CAD build for the part. Positions are in the model's coordinates, mm. Face numbers are marked on the shaded views. A direction names the side the tool comes from. Round coordinates to 2 decimals unless told otherwise and drop trailing zeros. Write each loop counter-clockwise with the first axis right and the second up, starting at its lowest first coordinate (ties: lowest second). Pieces come first, ordered by that corner, then holes. Notation, with made-up numbers: (51.5, 66) - (66.5, 66) arc R29 cw to (66.5, 90) - close; hole circle Ø8 at (13, 1). An arc over 180 degrees is marked (long way). Answer in a Markdown table with one row per item.
```python
from build123d import *

# Parameters (mm, degrees)
SKETCH1_W           = 20
SKETCH1_H           = 27
SKETCH1_R           = 2.5
BOSS_EXTRUDE1_DEPTH = 3
SKETCH2_W           = 3
SKETCH2_H           = 27
BOSS_EXTRUDE2_DEPTH = 15
SKETCH3_R           = 4
CUT_EXTRUDE1_DEPTH  = 15
CHAMFER1_SIZE       = 2


with BuildPart() as part:
    # Sketch1 → Boss-Extrude1 (new body)
    with BuildSketch(Plane(origin=(0, 0, 0), x_dir=(0, 0, -1), z_dir=(1, 0, 0))):
        with Locations((10, 13.5)):
            Rectangle(SKETCH1_W, SKETCH1_H)
        with Locations((10, 7)):
            Circle(SKETCH1_R, mode=Mode.SUBTRACT)
        with Locations((10, 20)):
            Circle(SKETCH1_R, mode=Mode.SUBTRACT)
    extrude(amount=BOSS_EXTRUDE1_DEPTH)

    # Sketch2 → Boss-Extrude2 (add)
    with BuildSketch(Plane(origin=(3, 0, 0), x_dir=(0, 0, -1), z_dir=(1, 0, 0))):
        with Locations((18.5, 13.5)):
            Rectangle(SKETCH2_W, SKETCH2_H)
    extrude(amount=BOSS_EXTRUDE2_DEPTH)

    # Sketch3 → Cut-Extrude1 (cut)
    with BuildSketch(Plane(origin=(0, 0, -20), x_dir=(-1, 0, 0), z_dir=(0, 0, -1))):
        with Locations((-10.5, 19.75)):
            Circle(SKETCH3_R)
        with Locations((-10.5, 7.25)):
            Circle(SKETCH3_R)
    extrude(amount=-CUT_EXTRUDE1_DEPTH, mode=Mode.SUBTRACT)

    # Chamfer1
    chamfer1_edges = [part.edges().sort_by_distance(p)[0] for p in [
        (18, 27, -18.5),
        (18, 0, -18.5),
    ]]
    chamfer(chamfer1_edges, length=CHAMFER1_SIZE)


solid = part.part
```
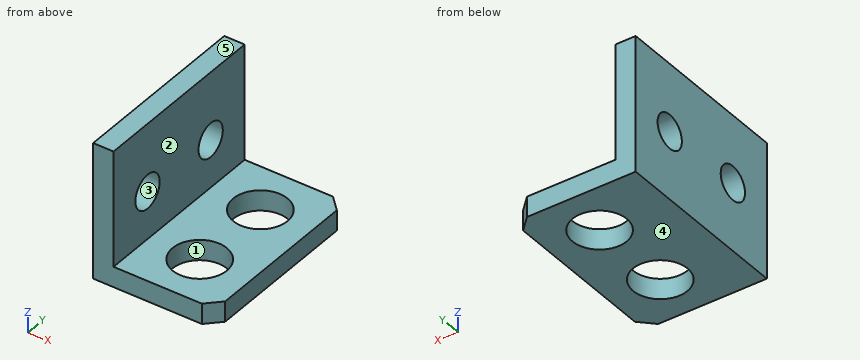
Q1. Saw through at C-C on z = -18.5. List the corners of the cut face in (x, y).
Computed:
| item | result |
|---|---|
| outline | (0, 0) - (16, 0) - (18, 2) - (18, 25) - (16, 27) - (0, 27) - close; hole circle Ø8 at (10.5, 7.25); hole circle Ø8 at (10.5, 19.75) |
Q2. Drill centre lines: line 1 (Y direction, x = 0.6, z = -10); line 2 (Y direction, x = 10.5, z = -18.15); line 3 (X direction, y = 21.25, z = -15). Where is each one in solid material? Low to high.
Computed:
| item | result |
|---|---|
| line 1 | y = 0 to 4.5, 9.5 to 17.5, 22.5 to 27 |
| line 2 | y = 0 to 3.25, 11.25 to 15.75, 23.75 to 27 |
| line 3 | x = 0 to 3 |
Q3. Saw through at B-B on x = 1.5. List the corners of the cut face in (y, z).
Computed:
| item | result |
|---|---|
| outline | (0, -20) - (27, -20) - (27, 0) - (0, 0) - close; hole circle Ø5 at (7, -10); hole circle Ø5 at (20, -10) |
Q4. 3-axis set-ups, long thin cutter, end or side, ignore diameter. For the marked faces 1 and 2: which of +Z, -Z, +X, -X, +Y, -Y reach the whole face in a straight line?
Computed:
| item | result |
|---|---|
| face 1 | +Z, -Z |
| face 2 | +Z, +X, +Y, -Y |
Q5. Flat gauge pins, fed straight in: pin 1 (8.5 mm diameter, centred on y = 17.5, z = -8, fed in from +X); pin 2 (5 mm diameter, centred on x = 15.5, y = 4.5, fed in from +Z). Where does each tip first touch, or does it go through?
Computed:
| item | result |
|---|---|
| pin 1 | stops at x = 3 |
| pin 2 | stops at z = -17 |
Q6. Saw through at D-D on x = 10.5. List the corners of the cut face in (y, z), then the cut area to 3 significant figures.
Computed:
| item | result |
|---|---|
| outline | (0, -20) - (3.25, -20) - (3.25, -17) - (0, -17) - close; (11.25, -20) - (15.75, -20) - (15.75, -17) - (11.25, -17) - close; (23.75, -20) - (27, -20) - (27, -17) - (23.75, -17) - close |
| area | 33.0 mm2 |
Q7. Pull direction Z, two halves, no side cores. Call the marked faces 3, 4 and 5: released by +Z, released by -Z, zero draft, split by the parting line, or undercut.
Computed:
| item | result |
|---|---|
| face 3 | undercut |
| face 4 | released by -Z |
| face 5 | released by +Z |
Q8. Saw through at A-A on z = -12. List the corners of the cut face in (x, y).
Computed:
| item | result |
|---|---|
| outline | (0, 0) - (3, 0) - (3, 5.5) - (0, 5.5) - close; (0, 8.5) - (3, 8.5) - (3, 18.5) - (0, 18.5) - close; (0, 21.5) - (3, 21.5) - (3, 27) - (0, 27) - close |
